Geometry check sheet. Reference: the model listing, model coordinates, mm. Face numbers are marked on the shaded views. A direction names the side the tool comes from. Round coordinates to 2 decimals unless told otherwise and drop trailing zeros. Order: outer loops, then holes, each group sorted by start corner. A loop starts at its lowest first (then second) coordinate and runs counter-clockwise, first axis right, second up. Notation, with made-up numbers: (14, 89.5) -> (22, 89.5) arc R12 ccw to (22, 110.5) -> close; hole circle Ø1 at (19.25, -23.75). An arc over 180 degrees is marked (long way). Use a Markdown table: item, result. Add a question column.
Item 1: Set-up check for the marked faces 1, 2 and 3: record each of +Z, -Z, +X, -X, +Y, -Y from which the full face is reachable in a straight line by a thin tool's end or side.
Item 2: Sectioned sample at D-D, the plane x = 9.5. Record the cut outline in (y, z).
Item 3: Gauge pin test, flat ends, axial feed: pin 1 Ø10 at (x, z) = (7, 6) entering from +Y; pin 2 Ø3 at (x, y) = (-0.5, -109.5) entering from -Z; pin 3 Ø10 at (y, z) = (-54.5, 0.5) entering from +X. Record the tip position at first contact, or that the pin passes through.
Item 4: Sectioned sample at C-C, the plane y = -13.5. Record the cut outline in (x, z), and give its area (3 significant figures).
Item 5: Material ranges on probe 1 along Y at (x, z) = (-22, 10); probe 2 along Z at (x, y) = (-3, -103.5); probe 3 along X at (y, z) = (-56, -1), recorded low to high. Write a range as [from, to].
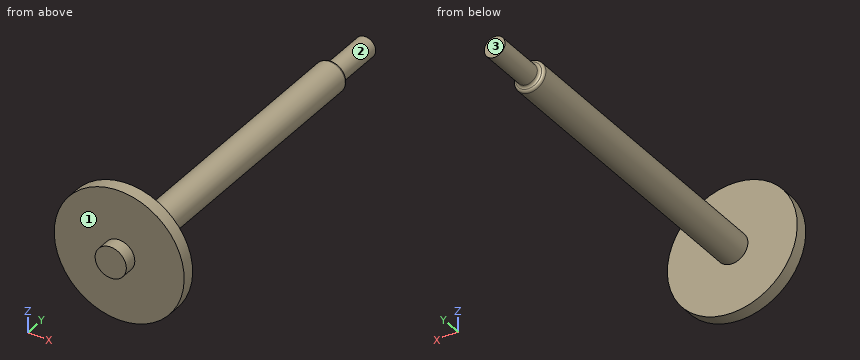
from build123d import *

# Parameters (mm, degrees)
SKETCH1_R           = 4
BOSS_EXTRUDE1_DEPTH = 10
SKETCH2_R           = 6
BOSS_EXTRUDE2_DEPTH = 120
SKETCH3_R           = 25
BOSS_EXTRUDE3_DEPTH = 5
SKETCH4_R           = 6
BOSS_EXTRUDE4_DEPTH = 5
FILLET2_R           = 1


with BuildPart() as part:
    # Sketch1 → Boss-Extrude1 (new, symmetric)
    with BuildSketch(Plane(origin=(0, 0, 0), x_dir=(1, 0, 0), z_dir=(0, 1, 0))):
        with Locations(Location((0, 0, 0), (0, 0, 270))):
            Circle(SKETCH1_R)
    extrude(amount=BOSS_EXTRUDE1_DEPTH, both=True)

    # Sketch2 → Boss-Extrude2 (add)
    with BuildSketch(Plane.XZ.offset(10)):
        with Locations(Location((0, 0, 0), (0, 0, 270))):
            Circle(SKETCH2_R)
    extrude(amount=BOSS_EXTRUDE2_DEPTH)

    # Sketch3 → Boss-Extrude3 (add)
    with BuildSketch(Plane.XZ.offset(130)):
        with Locations(Location((0, 0, 0), (0, 0, 270))):
            Circle(SKETCH3_R)
    extrude(amount=BOSS_EXTRUDE3_DEPTH)

    # Sketch4 → Boss-Extrude4 (add)
    with BuildSketch(Plane.XZ.offset(135)):
        with Locations(Location((0, 0, 0), (0, 0, 270))):
            Circle(SKETCH4_R)
    extrude(amount=BOSS_EXTRUDE4_DEPTH)

    # Fillet2
    fillet2_edges = [part.edges().sort_by_distance(p)[0] for p in [
        (0, -10, -4),
        (0, -10, 6),
    ]]
    fillet(fillet2_edges, radius=FILLET2_R - 0.0001)  # a hair under: the kernel refuses the full size


solid = part.part
Found:
| question | item | result |
|---|---|---|
| 1 | face 1 | -Y |
| 1 | face 2 | +Y |
| 1 | face 3 | +Z, -Z, +X, -X, +Y |
| 2 | outline | (-135, -23.12) -> (-130, -23.12) -> (-130, 23.12) -> (-135, 23.12) -> close |
| 3 | pin 1 | stops at y = -9.63 |
| 3 | pin 2 | stops at z = -6 |
| 3 | pin 3 | stops at x = 6 |
| 4 | outline | circle Ø12 at (0, 0) |
| 4 | area | 113 mm2 |
| 5 | probe 1 | y = [-135, -130] |
| 5 | probe 2 | z = [-5.2, 5.2] |
| 5 | probe 3 | x = [-5.92, 5.92] |
